Here's the drawing with two shaded views (mm, measured from the low corner). I have some questions. Round coordinates to 2 decimals unless told otherwise and drop trailing zeros. Write each loop counter-clockwise with the first axis right and the second up, starting at its lowest first coordinate (ties: lowest second). Pieces come first, ordered by that corner, then holes. Notation, with made-up numbers: (-25, -19.75) -> (-5, -19.75) arc R24 ccw to (-5, -7.75) -> close; hole circle Ø2 at (58.25, -32.75). An arc over 180 degrees is marked (long way). Use CSV: the item, a comma, the result in double quotes.
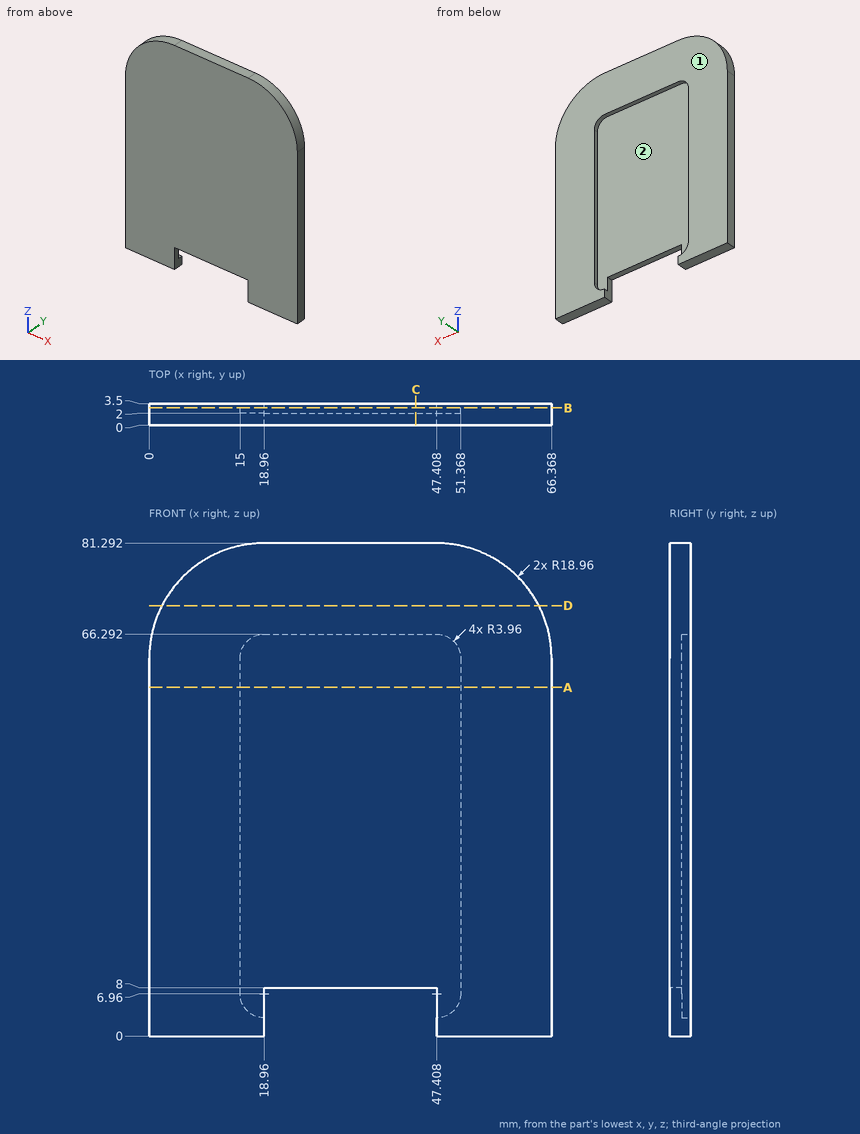
Q1. Suppose I cut it at D-D (z = 71). Write out the boundary of the cut face in (x, y).
Resolved:
outline,"(2.1, 0) -> (64.27, 0) -> (64.27, 3.5) -> (2.1, 3.5) -> close"
Q2. Suppose I cut it at B-B (y = 2.85). Write out the boundary of the cut face in (x, z), and give its area (3 significant figures).
Resolved:
outline,"(0, 0) -> (18.96, 0) -> (18.96, 3) arc R3.96 cw to (15, 6.96) -> (15, 62.33) arc R3.96 cw to (18.96, 66.29) -> (47.41, 66.29) arc R3.96 cw to (51.37, 62.33) -> (51.37, 6.96) arc R3.96 cw to (47.41, 3) -> (47.41, 0) -> (66.37, 0) -> (66.37, 62.33) arc R18.96 ccw to (47.41, 81.29) -> (18.96, 81.29) arc R18.96 ccw to (0, 62.33) -> close"
area,"2,870 mm^2"
Q3. Will these pins go through, and if not, where does the flat tip stop? P1, Ø2, axis at x = 59, y = 2, coming from the +Z side; P2, Ø1, axis at x = 38.5, y = 1.5, coming from the -Z side.
Resolved:
P1,"stops at z = 78.06"
P2,"stops at z = 8"
Q4. Suppose I cut it at C-C (x = 44). Write out the boundary of the cut face in (y, z), and give its area (3 significant figures).
Resolved:
outline,"(0, 8) -> (2, 8) -> (2, 66.29) -> (3.5, 66.29) -> (3.5, 81.29) -> (0, 81.29) -> close"
area,"169 mm^2"
Q5. Please list where these lines run through material, in increasing order: probe 1 along X at (y, z) = (2.8, 54); probe 2 along Z at (x, y) = (20.5, 1.55); probe 3 along Z at (x, y) = (36, 2.25).
Resolved:
probe 1,"x = 0 to 15, 51.37 to 66.37"
probe 2,"z = 8 to 81.29"
probe 3,"z = 66.29 to 81.29"
Q6. Suppose I cut it at A-A (z = 57.5). Write out the boundary of the cut face in (x, y), and give its area (3 significant figures).
Resolved:
outline,"(0, 0) -> (66.37, 0) -> (66.37, 3.5) -> (51.37, 3.5) -> (51.37, 2) -> (15, 2) -> (15, 3.5) -> (0, 3.5) -> close"
area,"178 mm^2"
Q7. If we mould it in two halves opening along Z, with no side actions, what happens to the marked faces 1 and 2? For each: released by +Z, released by -Z, zero draft, split by the parting line, or undercut.
Resolved:
face 1,"zero draft"
face 2,"undercut"
